Part print with two shaded views. Sizes in mm from the minimum x, y, z corner. Round coordinates to 2 decimals unless told otherwise and drop trailing zeros. Loops run counter-clockwise (first coordinate to the right, second up) from the corner with the lowest first, then second, coordinate; pieces in that order, holes last.
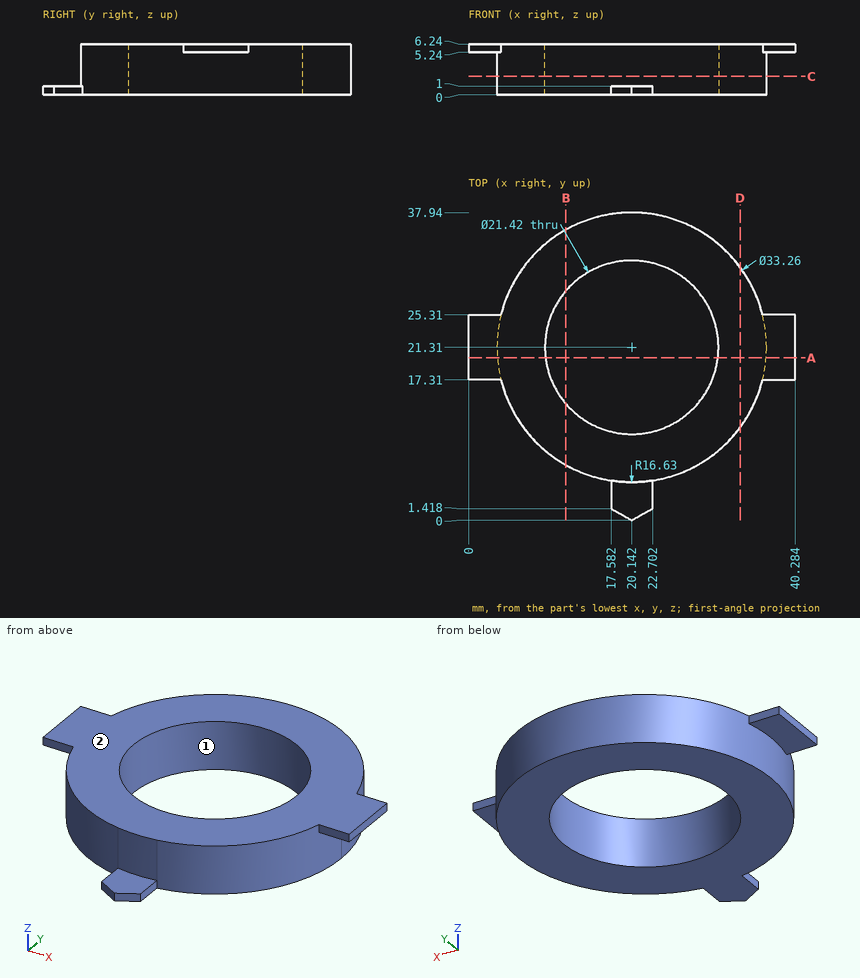
Item 1: Cut at B-B (x = 12). List the corners of the cut face in (y, z).
Verdict:
outline: (6.81, 0) - (14.35, 0) - (14.35, 6.24) - (6.81, 6.24) - close; (28.27, 0) - (35.81, 0) - (35.81, 6.24) - (28.27, 6.24) - close
Item 2: Cut at D-D (x = 33.5). List the corners of the cut face in (y, z) (1 decimal).
Verdict:
outline: (11.4, 0) - (31.2, 0) - (31.2, 6.2) - (11.4, 6.2) - close
Item 3: Cut at A-A (y = 20). List the corners of the cut face in (x, z).
Verdict:
outline: (0, 5.24) - (3.56, 5.24) - (3.56, 0) - (9.51, 0) - (9.51, 6.24) - (0, 6.24) - close; (30.77, 0) - (36.72, 0) - (36.72, 5.24) - (40.28, 5.24) - (40.28, 6.24) - (30.77, 6.24) - close
Item 4: Wall check: L1, parallel to Y at x = 19.5, z = 4.75; L2, parallel to Y at x = 23, z = 3.5; L3, parallel to X at y = 17, z = 2.25 (1 decimal). Give the ranges that are in metal, low to high.
Verdict:
L1: y = 4.69 to 10.62, 32 to 37.93
L2: y = 4.93 to 10.99, 31.63 to 37.69
L3: x = 4.1 to 10.3, 29.9 to 36.2
Item 5: Flat gauge pins, fed straight in: P1, Ø5.5, axis at x = 19.5, y = 2.5, coming from the +Z side; P2, Ø0.5, axis at y = 4, z = 0.5, coming from the -X side; P3, Ø3, axis at x = 10.5, z = 1, coming from the +Y side; P4, Ø0.5, axis at y = 3.5, z = 0.5, coming from the +X side. Where does each tip first touch, or does it go through?
Verdict:
P1: stops at z = 6.24
P2: stops at x = 17.58
P3: stops at y = 35.81
P4: stops at x = 22.7
Item 6: Mould opens along Y. For the marked faces 1 and 2 say: released by +Y, released by -Y, zero draft, split by the parting line, or undercut.
Verdict:
face 1: undercut
face 2: zero draft
Item 7: Cut at C-C (z = 2.25). List the corners of the cut face in (x, y).
Verdict:
outline: circle Ø33.26 at (20.14, 21.31); hole circle Ø21.42 at (20.14, 21.31)
